Model file for the job. Use its own axes, mm. A direction names the side the tool comes from. Round coordinates to 2 decimals unless told otherwise and drop trailing zeros. Loops run counter-clockwise (first coordinate to the right, second up) from the corner with the lowest first, then second, coordinate; pieces in that order, holes last. Notation, with made-up numbers: (-20, 4.5) -> (30, 4.5) arc R15 ccw to (30, 28.5) -> close; hole circle Ø3 at (69.5, 72.25). An arc over 180 degrees is marked (long way). Use a Markdown table: item, result.
from build123d import *

# Parameters (mm, degrees)
MODEL_R                 = 6
MODEL_R_2               = 8
SALIENTE_EXTRUIR1_DEPTH = 3


with BuildPart() as part:
    # Model → Saliente-Extruir1 (new body)
    with BuildSketch(Plane.XY):
        with BuildLine():
            Line((52.149227215, 40.252), (52.149227215, 37.252))
            ThreePointArc((52.149227215, 37.252), (52.442120434, 36.544893219), (53.149227215, 36.252))
            Line((53.149227215, 36.252), (61.149227215, 36.252))
            ThreePointArc((61.149227215, 36.252), (61.856333997, 35.959106781), (62.149227215, 35.252))
            Line((62.149227215, 35.252), (62.149227215, 12.636622367))
            Line((62.149227215, 12.636622367), (62.149227215, -18.748))
            ThreePointArc((62.149227215, -18.748), (61.856333997, -19.455106781), (61.149227215, -19.748))
            Line((61.149227215, -19.748), (53.149227215, -19.748))
            ThreePointArc((53.149227215, -19.748), (52.442120434, -20.040893219), (52.149227215, -20.748))
            Line((52.149227215, -20.748), (52.149227215, -42.748))
            ThreePointArc((52.149227215, -42.748), (51.856333997, -43.455106781), (51.149227215, -43.748))
            Line((51.149227215, -43.748), (40.985615848, -43.748))
            Line((40.985615848, -43.748), (40.985615848, -39.748))
            Line((40.985615848, -39.748), (37.985615848, -39.748))
            Line((37.985615848, -39.748), (37.985615848, -43.748))
            Line((37.985615848, -43.748), (34.985615848, -43.748))
            ThreePointArc((34.985615848, -43.748), (34.278509066, -43.455106781), (33.985615848, -42.748))
            Line((33.985615848, -42.748), (33.985615848, -20.748))
            ThreePointArc((33.985615848, -20.748), (33.692722629, -20.040893219), (32.985615848, -19.748))
            Line((32.985615848, -19.748), (24.985615848, -19.748))
            ThreePointArc((24.985615848, -19.748), (24.278509066, -20.040893219), (23.985615848, -20.748))
            Line((23.985615848, -20.748), (23.985615848, -42.748))
            ThreePointArc((23.985615848, -42.748), (23.692722629, -43.455106781), (22.985615848, -43.748))
            Line((22.985615848, -43.748), (19.985615848, -43.748))
            Line((19.985615848, -43.748), (19.985615848, -39.748))
            Line((19.985615848, -39.748), (16.985615848, -39.748))
            Line((16.985615848, -39.748), (16.985615848, -43.748))
            Line((16.985615848, -43.748), (6.82200448, -43.748))
            ThreePointArc((6.82200448, -43.748), (6.114897699, -43.455106781), (5.82200448, -42.748))
            Line((5.82200448, -42.748), (5.82200448, -20.969725915))
            ThreePointArc((5.82200448, -20.969725915), (5.529111261, -20.262619134), (4.82200448, -19.969725915))
            Line((4.82200448, -19.969725915), (-3.17799552, -19.969725915))
            ThreePointArc((-3.17799552, -19.969725915), (-3.885102301, -19.676832696), (-4.17799552, -18.969725915))
            Line((-4.17799552, -18.969725915), (-4.17799552, 14.641137042))
            Line((-4.17799552, 14.641137042), (-4.17799552, 35.252))
            ThreePointArc((-4.17799552, 35.252), (-3.885102301, 35.959106781), (-3.17799552, 36.252))
            Line((-3.17799552, 36.252), (4.82200448, 36.252))
            ThreePointArc((4.82200448, 36.252), (5.529111261, 36.544893219), (5.82200448, 37.252))
            Line((5.82200448, 37.252), (5.82200448, 40.252))
            ThreePointArc((5.82200448, 40.252), (5.529111261, 40.959106781), (4.82200448, 41.252))
            Line((4.82200448, 41.252), (1.82200448, 41.252))
            ThreePointArc((1.82200448, 41.252), (1.114897699, 41.544893219), (0.82200448, 42.252))
            Line((0.82200448, 42.252), (0.82200448, 45.252))
            ThreePointArc((0.82200448, 45.252), (0.529111261, 45.959106781), (-0.17799552, 46.252))
            Line((-0.17799552, 46.252), (-3.17799552, 46.252))
            ThreePointArc((-3.17799552, 46.252), (-3.885102301, 46.544893219), (-4.17799552, 47.252))
            Line((-4.17799552, 47.252), (-4.17799552, 85.252))
            ThreePointArc((-4.17799552, 85.252), (-4.470888739, 85.959106781), (-5.17799552, 86.252))
            Line((-5.17799552, 86.252), (-8.67799552, 86.252))
            Line((-8.67799552, 86.252), (-13.17799552, 86.252))
            ThreePointArc((-13.17799552, 86.252), (-13.885102301, 86.544893219), (-14.17799552, 87.252))
            Line((-14.17799552, 87.252), (-14.17799552, 104.252))
            ThreePointArc((-14.17799552, 104.252), (-13.592209082, 105.666213562), (-12.17799552, 106.252))
            Line((-12.17799552, 106.252), (3.82200448, 106.252))
            ThreePointArc((3.82200448, 106.252), (5.236218042, 105.666213562), (5.82200448, 104.252))
            Line((5.82200448, 104.252), (5.82200448, 97.252))
            ThreePointArc((5.82200448, 97.252), (6.114897699, 96.544893219), (6.82200448, 96.252))
            Line((6.82200448, 96.252), (49.82200448, 96.252))
            ThreePointArc((49.82200448, 96.252), (50.529111261, 96.544893219), (50.82200448, 97.252))
            Line((50.82200448, 97.252), (50.82200448, 104.252))
            ThreePointArc((50.82200448, 104.252), (51.407790918, 105.666213562), (52.82200448, 106.252))
            Line((52.82200448, 106.252), (68.82200448, 106.252))
            ThreePointArc((68.82200448, 106.252), (70.236218042, 105.666213562), (70.82200448, 104.252))
            Line((70.82200448, 104.252), (70.82200448, 87.252))
            ThreePointArc((70.82200448, 87.252), (70.529111261, 86.544893219), (69.82200448, 86.252))
            Line((69.82200448, 86.252), (63.149227215, 86.252))
            ThreePointArc((63.149227215, 86.252), (62.442120434, 85.959106781), (62.149227215, 85.252))
            Line((62.149227215, 85.252), (62.149227215, 66.752))
            Line((62.149227215, 66.752), (62.149227215, 47.252))
            ThreePointArc((62.149227215, 47.252), (61.856333997, 46.544893219), (61.149227215, 46.252))
            Line((61.149227215, 46.252), (58.149227215, 46.252))
            ThreePointArc((58.149227215, 46.252), (57.442120434, 45.959106781), (57.149227215, 45.252))
            Line((57.149227215, 45.252), (57.149227215, 42.252))
            ThreePointArc((57.149227215, 42.252), (56.856333997, 41.544893219), (56.149227215, 41.252))
            Line((56.149227215, 41.252), (53.149227215, 41.252))
            ThreePointArc((53.149227215, 41.252), (52.442120434, 40.959106781), (52.149227215, 40.252))
        make_face()
        with Locations((28.532877275, 62.00057999)):
            Circle(MODEL_R, mode=Mode.SUBTRACT)
        with Locations((41.532877275, 81.20057999)):
            Circle(MODEL_R_2, mode=Mode.SUBTRACT)
        with Locations((15.532877275, 81.20057999)):
            Circle(MODEL_R_2, mode=Mode.SUBTRACT)
        Polygon((12.985615848, 18.252), (29.485615848, 18.252), (44.985615848, 18.252), (44.985615848, -13.748), (12.985615848, -13.748), align=None, mode=Mode.SUBTRACT)
        with BuildLine():
            Line((37.863153208, 48.00057999), (19.202601343, 48.00057999))
            ThreePointArc((19.202601343, 48.00057999), (18.250601998, 47.306680051), (18.619787227, 46.187974485))
            ThreePointArc((18.619787227, 46.187974485), (28.532877275, 43.00057999), (38.445967323, 46.187974485))
            ThreePointArc((38.445967323, 46.187974485), (38.815152552, 47.306680051), (37.863153208, 48.00057999))
        make_face(mode=Mode.SUBTRACT)
    extrude(amount=SALIENTE_EXTRUIR1_DEPTH)


solid = part.part
Q1. Band-saw the part on A-A, the plane y = 2. Give the cut face in (x, z).
Results list:
| item | result |
|---|---|
| outline | (-4.18, 0) -> (12.99, 0) -> (12.99, 3) -> (-4.18, 3) -> close; (44.99, 0) -> (62.15, 0) -> (62.15, 3) -> (44.99, 3) -> close |
Q2. Band-saw the part on D-D, the plane z = 1.9. Give the number of separate pieces and of enclosed holes in the cut face, plus the area to 3 significant figures.
Results list:
| item | result |
|---|---|
| separate pieces | 1 |
| enclosed holes | 5 |
| area | 7,360 mm² |
Q3. Flat gauge pins, fed straight in: pin 1 (1.5 mm diameter, centred on y = -42, z = 1.5, fed in from -X); pin 2 (1 mm diameter, centred on x = -2, y = 13.5, fed in from -Z); pin 3 (1.5 mm diameter, centred on y = -37, z = 1, fed in from +X); pin 4 (1.5 mm diameter, centred on x = 32.5, z = 1, fed in from -Y). Where does each tip first touch, or does it go through?
Results list:
| item | result |
|---|---|
| pin 1 | stops at x = 5.82 |
| pin 2 | stops at z = 0 |
| pin 3 | stops at x = 52.15 |
| pin 4 | stops at y = -19.78 |
Q4. Tool access for faces 1 (the face through (-9, 86.252, 1)), 2 (the face through (12.986, 2, 1)), 3 (the face through (5.822, 101, 1)): list every direction of +Z, -Z, +X, -X, +Y, -Y with a clear straight run to the whole face (end or side of a thin tool).
Results list:
| item | result |
|---|---|
| face 1 | +Z, -Z, -X, -Y |
| face 2 | +Z, -Z |
| face 3 | +Z, -Z, +Y |
Q5. Drill centre lines: L1, parallel to Y at x = 28.5, z = 0.85; L2, parallel to X at y = 0, z = 1.35; L3, parallel to Y at x = 26.5, z = 2.05. Where is each one in solid material? Low to high. Write a range as from..to.
Results list:
| item | result |
|---|---|
| L1 | y = -19.75..-13.75, 18.25..43, 48..56, 68..96.25 |
| L2 | x = -4.18..12.99, 44.99..62.15 |
| L3 | y = -19.75..-13.75, 18.25..43.12, 48..56.36, 67.65..96.25 |
Q6. Pull direction Y, two halves, no side cores. Call faces 4 (the face through (-14.178, 96, 1)), 5 (the face through (1, -19.97, 1)), 6 (the face through (28.4, 43, 1.5)): released by +Y, released by -Y, zero draft, split by the parting line, or undercut.
Results list:
| item | result |
|---|---|
| face 4 | zero draft |
| face 5 | released by -Y |
| face 6 | undercut |
Q7. Band-saw the part on C-C, the plane x = 10.5. Give the cut face in (y, z), plus the area to 3 significant figures.
Results list:
| item | result |
|---|---|
| outline | (-43.75, 0) -> (74.98, 0) -> (74.98, 3) -> (-43.75, 3) -> close; (87.42, 0) -> (96.25, 0) -> (96.25, 3) -> (87.42, 3) -> close |
| area | 383 mm² |
Q8. Band-saw the part on B-B, the plane y = 75. Give the cut face in (x, z).
Results list:
| item | result |
|---|---|
| outline | (-4.18, 0) -> (10.48, 0) -> (10.48, 3) -> (-4.18, 3) -> close; (20.59, 0) -> (36.48, 0) -> (36.48, 3) -> (20.59, 3) -> close; (46.59, 0) -> (62.15, 0) -> (62.15, 3) -> (46.59, 3) -> close |
